Geometry check sheet. Reference: drawing and pictorial views, mm from the part's lowest x, y, z. Round coordinates to 2 decimals unless told otherwise and drop trailing zeros. Loops run counter-clockwise (first coordinate to the right, second up) from the corner with the lowest first, then second, coordinate; pieces in that order, holes last. Notation, with made-up numbers: (-5.5, 60) -> (36.5, 60) arc R16 cw to (36.5, 72) -> close; hole circle Ø1 at (45, 63.25). An arc over 180 degrees is marked (long way). Use one line per item in the form item = value.
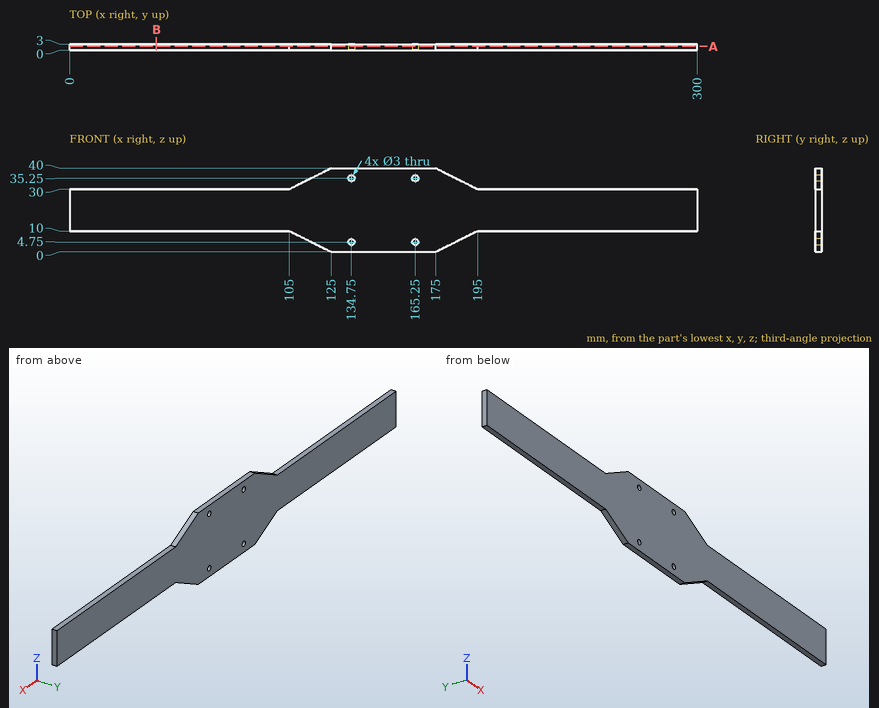
1. Gauge pin test, flat ends, axial feed: pin 1 (0.9 mm diameter, centred on x = 45, y = 2, fed in from -Z); pin 2 (3.5 mm diameter, centred on x = 165.25, z = 35.25, fed in from -Y); pin 3 (0.9 mm diameter, centred on x = 29.5, y = 1.5, fed in from +Z). Record the tip position at first contact, or that the pin passes through.
Return value:
pin_1 = 10
pin_2 = 0
pin_3 = 30
2. Section check B-B (x = 41.5). Record the boundary of the cut face in (y, z).
Return value:
outline = (0, 10) -> (3, 10) -> (3, 30) -> (0, 30) -> close
3. Material ranges on line 1 along Z through (x, y) = (134.75, 1.45); line 2 along X through (y, z) = (1.1, 4.75); line 3 along Z through (x, y) = (230.5, 2.4), recorded low to high.
Return value:
line_1 = 0 to 3.25, 6.25 to 33.75, 36.75 to 40
line_2 = 115.5 to 133.25, 136.25 to 163.75, 166.75 to 184.5
line_3 = 10 to 30
4. Section check A-A (y = 1.9). Record the boundary of the cut face in (x, z).
Return value:
outline = (0, 10) -> (105, 10) -> (125, 0) -> (175, 0) -> (195, 10) -> (300, 10) -> (300, 30) -> (195, 30) -> (175, 40) -> (125, 40) -> (105, 30) -> (0, 30) -> close; hole circle Ø3 at (134.75, 4.75); hole circle Ø3 at (134.75, 35.25); hole circle Ø3 at (165.25, 4.75); hole circle Ø3 at (165.25, 35.25)
